Can you work these out from the model? Positions are in its coordinate system, mm. Face numbers are marked on the shaded views. A direction names the side the tool comes from. Give positions to 0.01 mm unless a question says otherwise; leave off trailing zeros. Loops run counter-clockwise (first coordinate to the right, second up) from the corner with the lowest first, then second, coordinate; pieces in that order, holes last. Notation, with made-up numbers: (50, -4.75) -> (99, -4.75) arc R28 cw to (99, 32.25) -> close; hole circle Ø1 at (82.25, 0). An arc over 180 degrees is marked (long way). Return JSON: item names as keys, results as strings. Group by question number.
Q1. Suppose I cut it at D-D, the plane x = 21. Please give me the cut outline in (y, z).
Q2. Suppose I cut it at C-C, the plane z = -6.5. Please give me the cut outline in (x, y).
Q3. I need wall thicknesses on line 1 along X through (y, z) = (2, 0); line 2 along Y through (x, z) = (21, 3.25); line 3 along Z through (x, y) = (-15.5, 8.8). Which ranges of each line are inside material? Lowest first, please. Write a range as [from, to].
Q4. Suppose I cut it at A-A, the plane z = 0. Please give me the cut outline in (x, y), and give its area (3 significant figures).
Q5. Suppose I cut it at B-B, the plane x = 15.5. Please give me the cut outline in (y, z).
Q6. Which directions (+Z, -Z, +X, -X, +Y, -Y) give clear straight access to the entire face, cutting with the end or side of a thin tool? Please do the marked faces 4, 5 and 6.
Q7. Will these pins go through, and if not, where does the flat tip stop? pin 1 (4 mm diameter, centred on x = 21, y = 5, fed in from +Z); pin 2 (6.5 mm diameter, centred on x = -15.5, z = 0, fed in from +Y); pin 3 (2 mm diameter, centred on x = -19.5, y = 5.5, fed in from -Z).
Q8. Thinking about a two-plate mould opening in Z: for the marked faces 1, 2 and 3, which applies, pulls with the +Z half, pulls with the -Z half, needs draft (parallel to the pull), parting line crosses it, or undercut?
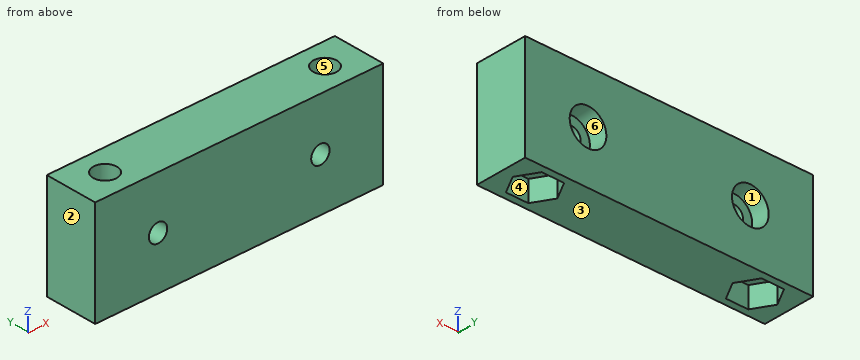
```python
from build123d import *

# Parameters (mm, degrees)
SKETCH1_W                                           = 55
SKETCH1_H                                           = 20
BOSS_EXTRUDE1_DEPTH                                 = 10
SKETCH2_R                                           = 2.25
CUT_EXTRUDE1_DEPTH                                  = 36.443617197
SKETCH3_R                                           = 1.75
CUT_EXTRUDE2_DEPTH                                  = 31.923292192
CBORE_FOR_M3_HEX_SOCKET_HEAD_CAP_SCREW1_D           = 3.4
CBORE_FOR_M3_HEX_SOCKET_HEAD_CAP_SCREW1_CBORE_D     = 7
CBORE_FOR_M3_HEX_SOCKET_HEAD_CAP_SCREW1_CBORE_DEPTH = 3.4
CUT_EXTRUDE3_DEPTH                                  = 4


with BuildPart() as part:
    # Sketch1 → Boss-Extrude1 (new body)
    with BuildSketch(Plane(origin=(0, 0, 0), x_dir=(1, 0, 0), z_dir=(0, 1, 0))):
        Rectangle(SKETCH1_W, SKETCH1_H)
    extrude(amount=BOSS_EXTRUDE1_DEPTH)

    # Sketch2 → Cut-Extrude1 (cut, through all)
    with BuildSketch(Plane.XY.offset(10)):
        with Locations((-21, 5)):
            Circle(SKETCH2_R)
        with Locations((21, 5)):
            Circle(SKETCH2_R)
    extrude(amount=-CUT_EXTRUDE1_DEPTH, mode=Mode.SUBTRACT)

    # Sketch3 → Cut-Extrude2 (cut, through all)
    with BuildSketch(Plane(origin=(0, 10, 0), x_dir=(1, 0, 0), z_dir=(0, 1, 0))):
        with Locations(Location((-15.5, 0, 0), (0, 0, 270))):
            Circle(SKETCH3_R)
        with Locations(Location((15.5, 0, 0), (0, 0, 270))):
            Circle(SKETCH3_R)
    extrude(amount=-CUT_EXTRUDE2_DEPTH, mode=Mode.SUBTRACT)

    # CBORE for M3 Hex Socket Head Cap Screw1 (through all)
    with Locations(Plane(origin=(0, 10, 0), x_dir=(1, 0, 0), z_dir=(0, 1, 0))):
        with Locations((-15.5, 0), (15.5, 0)):
            CounterBoreHole(CBORE_FOR_M3_HEX_SOCKET_HEAD_CAP_SCREW1_D / 2, CBORE_FOR_M3_HEX_SOCKET_HEAD_CAP_SCREW1_CBORE_D / 2, CBORE_FOR_M3_HEX_SOCKET_HEAD_CAP_SCREW1_CBORE_DEPTH)

    # Sketch6 → Cut-Extrude3 (cut)
    with BuildSketch(Plane(origin=(0, 0, -10), x_dir=(-1, 0, 0), z_dir=(0, 0, -1))):
        Polygon((-16.727608008, 5), (-18.863804004, 8.7), (-23.136195996, 8.7), (-25.272391992, 5), (-23.136195996, 1.3), (-18.863804004, 1.3), align=None)
        Polygon((16.727608008, 5), (18.863804004, 1.3), (23.136195996, 1.3), (25.272391992, 5), (23.136195996, 8.7), (18.863804004, 8.7), align=None)
    extrude(amount=-CUT_EXTRUDE3_DEPTH, mode=Mode.SUBTRACT)


solid = part.part
```
Ans:
{
 "1": {"outline": "(0, -10) -> (1.3, -10) -> (1.3, -6) -> (2.75, -6) -> (2.75, 10) -> (0, 10) -> close; (7.25, -6) -> (8.7, -6) -> (8.7, -10) -> (10, -10) -> (10, 10) -> (7.25, 10) -> close"},
 "2": {"outline": "(-27.5, 0) -> (27.5, 0) -> (27.5, 10) -> (-27.5, 10) -> close; hole (-25.27, 5) -> (-23.14, 1.3) -> (-18.86, 1.3) -> (-16.73, 5) -> (-18.86, 8.7) -> (-23.14, 8.7) -> close; hole (16.73, 5) -> (18.86, 1.3) -> (23.14, 1.3) -> (25.27, 5) -> (23.14, 8.7) -> (18.86, 8.7) -> close"},
 "3": {"line 1": "x = [-27.5, -17.25], [-13.75, 13.75], [17.25, 27.5]", "line 2": "y = [0, 2.75], [7.25, 10]", "line 3": "z = [-10, -3.5], [3.5, 10]"},
 "4": {"outline": "(-27.5, 0) -> (-17.25, 0) -> (-17.25, 6.6) -> (-19, 6.6) -> (-19, 10) -> (-27.5, 10) -> close; (-13.75, 0) -> (13.75, 0) -> (13.75, 6.6) -> (12, 6.6) -> (12, 10) -> (-12, 10) -> (-12, 6.6) -> (-13.75, 6.6) -> close; (17.25, 0) -> (27.5, 0) -> (27.5, 10) -> (19, 10) -> (19, 6.6) -> (17.25, 6.6) -> close; hole circle Ø4.5 at (-21, 5); hole circle Ø4.5 at (21, 5)", "area": "424 mm^2"},
 "5": {"outline": "(0, -10) -> (10, -10) -> (10, -3.5) -> (6.6, -3.5) -> (6.6, -1.75) -> (0, -1.75) -> close; (0, 1.75) -> (6.6, 1.75) -> (6.6, 3.5) -> (10, 3.5) -> (10, 10) -> (0, 10) -> close"},
 "6": {"face 4": "-Z", "face 5": "+Z, -Z", "face 6": "+Y"},
 "7": {"pin 1": "passes through", "pin 2": "stops at y = 6.6", "pin 3": "stops at z = -6"},
 "8": {"face 1": "undercut", "face 2": "needs draft", "face 3": "pulls with the -Z half"}
}
